Read the model definition and answer for the solid it produces. Units are mm, in the model's axes. Face numbers are marked on the shaded views. A direction names the side the tool comes from. Coordinates: 2 decimals unless noted, no trailing zeros. Loops run counter-clockwise (first coordinate to the right, second up) from the corner with the lowest first, then second, coordinate; pieces in that order, holes last. Notation, with made-up numbers: M -8.75,30.5 L 1.25,30.5 A31 cw 1.25,56.5 Z; hole C -33.5,-12.5 d6. An arc over 180 degrees is marked long. Put each result on its own line as item: value.
from build123d import *

# Parameters (mm, degrees)
SKETCH1_R           = 14
SKETCH1_R_2         = 2.517260593
SKETCH1_R_3         = 1.762082415
BOSS_EXTRUDE1_DEPTH = 5
SKETCH4_W           = 12
SKETCH4_H           = 5
BOSS_EXTRUDE4_DEPTH = 5
SKETCH6_W           = 5
SKETCH6_H           = 15
BOSS_EXTRUDE5_DEPTH = 30
SKETCH8_R           = 10.75
CUT_EXTRUDE2_DEPTH  = 3
FILLET1_R           = 5
FILLET2_R           = 1


with BuildPart() as part:
    # Sketch1 → Boss-Extrude1 (new body)
    with BuildSketch(Plane(origin=(0, 0, 0), x_dir=(1, 0, 0), z_dir=(0, 1, 0))):
        with Locations(Location((0, 0, 0), (0, 0, 270))):
            Circle(SKETCH1_R)
        with Locations(Location((0, 0, 0), (0, 0, 270))):
            Circle(SKETCH1_R_2, mode=Mode.SUBTRACT)
        with Locations(Location((0, 7, 0), (0, 0, 270))):
            Circle(SKETCH1_R_3, mode=Mode.SUBTRACT)
        with Locations(Location((7, 0, 0), (0, 0, 270))):
            Circle(SKETCH1_R_3, mode=Mode.SUBTRACT)
        with Locations(Location((0, -7, 0), (0, 0, 270))):
            Circle(SKETCH1_R_3, mode=Mode.SUBTRACT)
        with Locations(Location((-7, 0, 0), (0, 0, 270))):
            Circle(SKETCH1_R_3, mode=Mode.SUBTRACT)
    extrude(amount=BOSS_EXTRUDE1_DEPTH)

    # Sketch4 → Boss-Extrude4 (add)
    with BuildSketch(Plane(origin=(0, 5, 0), x_dir=(1, 0, 0), z_dir=(0, 1, 0))):
        with Locations((16.071494653, 0)):
            Rectangle(SKETCH4_W, SKETCH4_H)
    extrude(amount=-BOSS_EXTRUDE4_DEPTH)

    # Sketch6 → Boss-Extrude5 (add)
    with BuildSketch(Plane.XZ):
        with Locations((19.571494653, 5)):
            Rectangle(SKETCH6_W, SKETCH6_H)
    extrude(amount=-BOSS_EXTRUDE5_DEPTH)

    # Sketch8 → Cut-Extrude2 (cut)
    with BuildSketch(Plane.XZ):
        with Locations(Location((0, 0, 0), (0, 0, 270))):
            Circle(SKETCH8_R)
    extrude(amount=-CUT_EXTRUDE2_DEPTH, mode=Mode.SUBTRACT)

    # Fillet1
    # the kernel refuses this fillet: 5 mm, written as the material it adds along each edge
    with BuildSketch(Plane(origin=(17.071494653, 5, 2.5), x_dir=(-1, 0, 0), z_dir=(0, -1, 0))) as fillet1_piece_1:
        with BuildLine():
            CenterArc((5, -4.700866603), FILLET1_R, 109.919316249, 70.080683751)
            Line((0, -4.700866603), (-0.1, -4.700866603))
            Line((-0.1, -4.700866603), (-0.1, 0))
            Line((-0.1, 0), (0, 0.1))
            ThreePointArc((0, 0.1), (1.648258669, 0.1), (3.262447686, 0.094017332))
            Line((3.262447686, 0.094017332), (3.296517339, 0))
        make_face()
    extrude(amount=5)

    # Fillet2
    fillet2_edges = [part.edges().sort_by_distance(p)[0] for p in [
        (13.774977314, 2.5, 2.5),
        (13.774977314, 2.5, -2.5),
    ]]
    fillet(fillet2_edges, radius=FILLET2_R)


solid = part.part
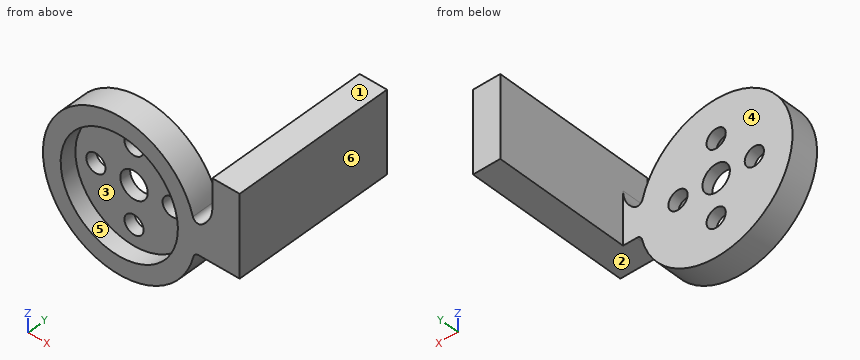
1) Which of the six approach directions +Z, -Z, +X, -X, +Y, -Y give full straight-line access (tool end or side, diameter ignored) to the marked faces 1, 2 and 3?
Answer list:
face 1: +Z, +X, +Y, -Y
face 2: -Z, +X, +Y, -Y
face 3: -Y
2) Find section C-C, the plane z = -7. Write down the section's boundary in (x, y).
Answer list:
outline: M -12.12,0 L -8.16,0 L -8.16,3 L -1.76,3 L -1.76,5 L -12.12,5 Z; M 1.76,3 L 8.16,3 L 8.16,0 L 12.12,0 L 12.12,5 L 1.76,5 Z
3) Find section D-D, the plane x = 6.5. Write down the section's boundary in (y, z), plus the area to 3 significant figures.
Answer list:
outline: M 0,-12.4 L 5,-12.4 L 5,-1.69 L 3,-1.69 L 3,-8.56 L 0,-8.56 Z; M 0,8.56 L 3,8.56 L 3,1.69 L 5,1.69 L 5,12.4 L 0,12.4 Z
area: 65.9 mm^2
4) Find section B-B, the plane x = 0. Write down the section's boundary in (y, z), plus the area to 3 significant figures.
Answer list:
outline: M 0,-14 L 5,-14 L 5,-8.76 L 3,-8.76 L 3,-10.75 L 0,-10.75 Z; M 0,10.75 L 3,10.75 L 3,8.76 L 5,8.76 L 5,14 L 0,14 Z; M 3,-5.24 L 5,-5.24 L 5,-2.52 L 3,-2.52 Z; M 3,2.52 L 5,2.52 L 5,5.24 L 3,5.24 Z
area: 51.3 mm^2
5) Determine the mould class of the marked faces 4, 5 and 6 for opening direction X: released by +X, released by -X, zero draft, split by the parting line, or undercut.
Answer list:
face 4: zero draft
face 5: undercut
face 6: released by +X
6) Given pin 1 Ø3 at (y, z) = (11, 8.5) entering from -X; pin 2 Ø4 at (x, z) = (11, -7) entering from +Y; pin 3 Ø5.5 at (x, y) = (19.5, 17) entering from +Z, each flat-ended and moving along its own axis, determine where each tip first touches the part or whether it passes through.
Answer list:
pin 1: stops at x = 17.07
pin 2: stops at y = 5
pin 3: stops at z = 12.5
7) Find section A-A, the plane z = 0. Write down the section's boundary in (x, y), plus the area to 3 significant figures.
Answer list:
outline: M -14,0 L -10.75,0 L -10.75,3 L -8.76,3 L -8.76,5 L -14,5 Z; M -5.24,3 L -2.52,3 L -2.52,5 L -5.24,5 Z; M 2.52,3 L 5.24,3 L 5.24,5 L 2.52,5 Z; M 8.76,3 L 10.75,3 L 10.75,0 L 22.07,0 L 22.07,30 L 17.07,30 L 17.07,5 L 8.76,5 Z
area: 217 mm^2
8) Straight lines are drawn through the part: line 1 (X direction, y = 4.3, z = 0); line 2 (X direction, y = 3.8, z = 7); line 3 (Z direction, x = 0, y = 4.1). For each, find the intervals that lie inside material, in ascending order. Write a range as [from, to].
Answer list:
line 1: x = [-14, -8.76], [-5.24, -2.52], [2.52, 5.24], [8.76, 22.07]
line 2: x = [-12.12, -1.76], [1.76, 12.12], [17.07, 22.07]
line 3: z = [-14, -8.76], [-5.24, -2.52], [2.52, 5.24], [8.76, 14]
